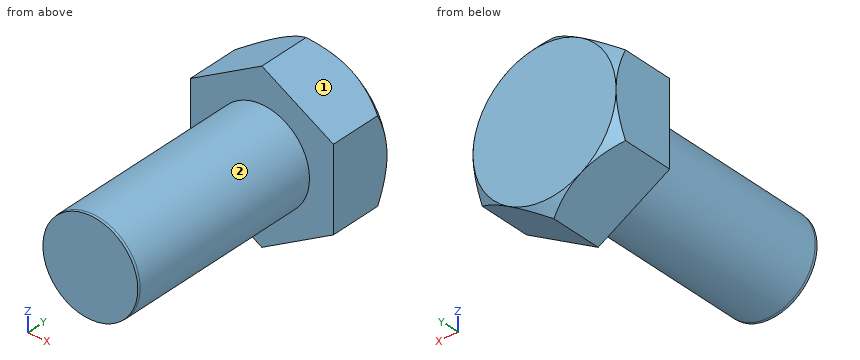
```python
from build123d import *

# Parameters (mm, degrees)
BOSS_EXTRUDE1_DEPTH = 6.35
SKETCH2_R           = 4.7625
BOSS_EXTRUDE2_DEPTH = 20.32
SKETCH3_OUTSIDE_W   = 63.834
SKETCH3_OUTSIDE_H   = 66.046
SKETCH3_OUTSIDE_R   = 7.1501
CUT_EXTRUDE1_DEPTH  = 20.32
CUT_EXTRUDE1_TAPER  = 45
CHAMFER1_SIZE       = 0.254
CHAMFER1_SIZE2      = 0.022222121


with BuildPart() as part:
    # Sketch1 → Boss-Extrude1 (new body)
    with BuildSketch(Plane(origin=(0, 0, 0), x_dir=(1, 0, 0), z_dir=(0, 1, 0))):
        Polygon((0, 8.256224319), (-7.1501, 4.12811216), (-7.1501, -4.12811216), (0, -8.256224319), (7.1501, -4.12811216), (7.1501, 4.12811216), align=None)
    extrude(amount=BOSS_EXTRUDE1_DEPTH)

    # Sketch2 → Boss-Extrude2 (add)
    with BuildSketch(Plane.XZ):
        Circle(SKETCH2_R)
    extrude(amount=BOSS_EXTRUDE2_DEPTH)

    # Sketch3 outside → Cut-Extrude1 (cut)
    with BuildSketch(Plane(origin=(0, 6.35, 0), x_dir=(1, 0, 0), z_dir=(0, 1, 0))):
        Rectangle(SKETCH3_OUTSIDE_W, SKETCH3_OUTSIDE_H)
        Circle(SKETCH3_OUTSIDE_R, mode=Mode.SUBTRACT)
    extrude(amount=-CUT_EXTRUDE1_DEPTH, taper=CUT_EXTRUDE1_TAPER, mode=Mode.SUBTRACT)

    # Chamfer1
    chamfer1_edges = [part.edges().sort_by_distance(p)[0] for p in [
        (-4.7625, -20.32, 0),
    ]]
    chamfer1_side = [part.faces().sort_by_distance(p)[0] for p in [
        (-4.7625, -10.16, 0),
    ]]
    chamfer(chamfer1_edges, length=CHAMFER1_SIZE, length2=CHAMFER1_SIZE2, reference=chamfer1_side[0])


solid = part.part
```
Can you work these out from the model? Positions are in its coordinate system, mm. Face numbers are marked on the shaded views. A direction names the side the tool comes from. Coordinates: 2 decimals unless noted, no trailing zeros. Loops run counter-clockwise (first coordinate to the right, second up) from the corner with the lowest first, then second, coordinate; pieces in that order, holes last. Notation, with made-up numbers: (-5, 42.25) -> (48, 42.25) arc R29 cw to (48, 73.25) -> close; hole circle Ø7 at (49, 82.25). An arc over 180 degrees is marked (long way). Put each result on its own line as item: value. Start each with the question number.
Q1. For the marked faces 1 and 2, which set-ups out of +Z, -Z, +X, -X, +Y, -Y let a thin tool reach every point of the face, with its end or its side?
Q2. I want a section at A-A (y = 1.75). Write out the boundary of the cut face in (x, z).
Q3. If I drill on line 1 (Y direction, x = 6.5, z = 1.5); line 2 (Z direction, x = 0, y = -6); line 3 (X direction, y = -17.75, z = -0.5), over which ranges is the centre line in solid material (lowest first)? Write a range as [from, to].
Q4. I want a section at B-B (y = -18.25). Write out the boundary of the cut face in (x, z) (1 decimal), plus the area to 3 significant figures.
Q5. I'm going to push flat-ended pins straight in: P1, Ø1, axis at y = -15, z = 1, coming from the -X side; P2, Ø4, axis at x = -2.5, y = -0.5, coming from the +Z side; P3, Ø5, axis at x = 4.5, y = 0, coming from the -Z side; P4, Ø6, axis at y = -2.5, z = 0, coming from the +X side. Where does each tip first touch, or does it pass through?
Taken from the geometry:
1. face 1: +Z, +X, +Y, -Y
1. face 2: -Y
2. outline: (-7.15, -4.13) -> (0, -8.26) -> (7.15, -4.13) -> (7.15, 4.13) -> (0, 8.26) -> (-7.15, 4.13) -> close
3. line 1: y = [0, 6.35]
3. line 2: z = [-4.76, 4.76]
3. line 3: x = [-4.74, 4.74]
4. outline: circle Ø9.5 at (0, 0)
4. area: 71.3 mm2
5. P1: stops at x = -4.74
5. P2: stops at z = 7.93
5. P3: stops at z = -7.1
5. P4: stops at x = 7.15
